Check sheet for the modelled part. Datum: model origin and axes. Units: mm. Face numbers are marked on the shaded views. Round coordinates to 2 decimals unless told otherwise and drop trailing zeros. Write each loop counter-clockwise with the first axis right and the second up, starting at its lowest first coordinate (ties: lowest second). Pieces come first, ordered by that corner, then holes. Notation, with made-up numbers: (-0.75, -37.5) - (16.25, -37.5) arc R18 cw to (16.25, -28.5) - close; hole circle Ø2 at (54, 11). An arc over 180 degrees is marked (long way). Answer as a JSON object with one key per item and string values. Group by question number.
Item 1: Release check for a two-part mould opening along Y. For the marked faces 1, 2 and 3 record: pulls with the +Y half, pulls with the -Y half, needs draft (parallel to the pull), parting line crosses it, or undercut.
Item 2: Sectioned sample at A-A on y = 12.7. Record the boundary of the cut face in (x, z).
Item 3: Thickness scan on line 1 (X direction, y = 28, z = 0.75); line 2 (Y direction, x = 0, z = 3.25); line 3 (X direction, y = 27, z = 0.45). Record the ranges inside material, lowest first.
Item 4: Sectioned sample at B-B on y = 25.4. Record the boundary of the cut face in (x, z) (3 decimals).
Item 5: Sectioned sample at D-D on x = 0. Record the boundary of the cut face in (y, z).
Item 6: Sectioned sample at C-C on z = 1. Record the boundary of the cut face in (x, y) (3 decimals).
Item 7: Gauge pin test, flat ends, axial feed: P1, Ø1, axis at x = -15, z = 3, coming from the -Y side; P2, Ø2, axis at y = 21.5, z = 2, coming from the +X side; P3, Ø3, axis at y = 21.5, z = 2.5, coming from the +X side. Record the tip position at first contact, or that the pin passes through.
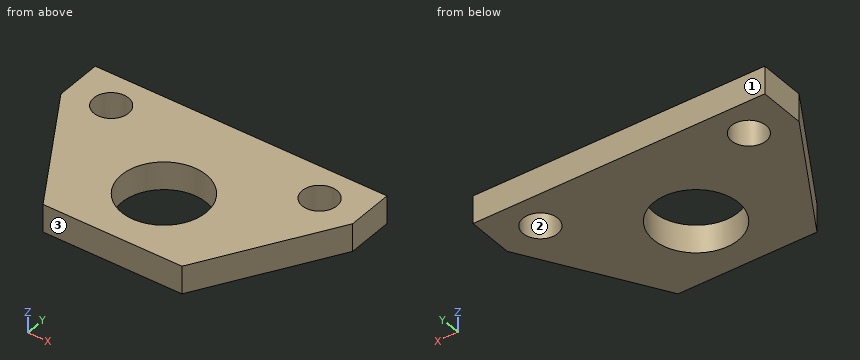
```python
from build123d import *

# Parameters (mm, degrees)
BOSS_EXTRUDE1_DEPTH = 5.08
SKETCH3_R           = 7.747
SKETCH3_R_2         = 3.175
CUT_EXTRUDE2_DEPTH  = 5.08


with BuildPart() as part:
    # Sketch1 → Boss-Extrude1 (new body)
    with BuildSketch(Plane.XY):
        Polygon((-31.75, 31.75), (31.75, 31.75), (12.7, 0), (-12.7, 0), align=None)
    extrude(amount=BOSS_EXTRUDE1_DEPTH)

    # Sketch3 → Cut-Extrude2 (cut)
    with BuildSketch(Plane.XY.offset(5.08)):
        with Locations((0, 12.7)):
            Circle(SKETCH3_R)
        with Locations((-19.05, 25.4)):
            Circle(SKETCH3_R_2)
        with Locations((19.05, 25.4)):
            Circle(SKETCH3_R_2)
        Polygon((-26.67, 23.283333333), (-26.67, 31.75), (-31.75, 31.75), align=None)
        Polygon((26.67, 31.75), (26.67, 23.283333333), (31.75, 31.75), align=None)
    extrude(amount=-CUT_EXTRUDE2_DEPTH, mode=Mode.SUBTRACT)


solid = part.part
```
Completed:
{
 "1": {"face 1": "pulls with the +Y half", "face 2": "undercut", "face 3": "pulls with the -Y half"},
 "2": {"outline": "(-20.32, 0) - (-7.75, 0) - (-7.75, 5.08) - (-20.32, 5.08) - close; (7.75, 0) - (20.32, 0) - (20.32, 5.08) - (7.75, 5.08) - close"},
 "3": {"line 1": "-26.67 to -20.87, -17.23 to 17.23, 20.87 to 26.67", "line 2": "0 to 4.95, 20.45 to 31.75", "line 3": "-26.67 to -21.79, -16.31 to 16.31, 21.79 to 26.67"},
 "4": {"outline": "(-26.67, 0) - (-22.225, 0) - (-22.225, 5.08) - (-26.67, 5.08) - close; (-15.875, 0) - (15.875, 0) - (15.875, 5.08) - (-15.875, 5.08) - close; (22.225, 0) - (26.67, 0) - (26.67, 5.08) - (22.225, 5.08) - close"},
 "5": {"outline": "(0, 0) - (4.95, 0) - (4.95, 5.08) - (0, 5.08) - close; (20.45, 0) - (31.75, 0) - (31.75, 5.08) - (20.45, 5.08) - close"},
 "6": {"outline": "(-26.67, 23.283) - (-12.7, 0) - (12.7, 0) - (26.67, 23.283) - (26.67, 31.75) - (-26.67, 31.75) - close; hole circle Ø6.35 at (-19.05, 25.4); hole circle Ø15.494 at (0, 12.7); hole circle Ø6.35 at (19.05, 25.4)"},
 "7": {"P1": "y = 3", "P2": "x = 26.2", "P3": "x = 26.5"}
}
